Verification items for the finished model (mm, model axes). A direction names the side the tool comes from. Coordinates: 2 decimals unless noted, no trailing zeros. Loops run counter-clockwise (first coordinate to the right, second up) from the corner with the lowest first, then second, coordinate; pieces in that order, holes last. Notation, with made-up numbers: (-36.75, -23) - (-13.75, -23) arc R23 ccw to (-13.75, 1) - close; hole circle Ø6 at (6, 18). An arc over 180 degrees is marked (long way). Answer as CSV lines item,"result". Start each with the question number.
1. Gauge pin test, flat ends, axial feed: P1, Ø12.5, axis at y = 170, z = 0, coming from the -X side; P2, Ø5, axis at x = 5, z = -399, coming from the +Y side. Record the tip position at first contact, or that the pin passes through.
2. Material ranges on line 1 (Y direction, x = 4.5, z = 184); line 2 (Z direction, x = 7.75, y = 550); line 3 (Z direction, x = 0.5, y = 189.5), recorded low to high. Write a range as [from, to].
3. Release check for a two-part mould opening along Z. For faces 3 (the flat face through (0, 81, -130)), 4 (the flat face through (4.93, 261.39, -14.83)), 5 (the flat face through (4.93, 177.45, -246.5)) record: pulls with the +Z half, pulls with the -Z half, needs draft (parallel to the pull), parting line crosses it, or undercut.
4. Cross-section at C-C (z = -301). Enter the section's corners in (x, y), plus the area to 3 significant figures.
5. Cross-section at B-B (x = 1.75). State how many separate pieces and enclosed holes the cut face has, plus the area to 3 significant figures.
6. Set-up check for faces 1 (the flat face through (4.93, 63.37, 210.65)), 2 (the flat face through (10, 81, -130)): record each of +Z, -Z, +X, -X, +Y, -Y from which the full face is reachable in a straight line by a thin tool's end or side.
7. Cross-section at A-A (y = 251.5). Enter the section's corners in (x, z).
8. Cross-section at D-D (y = 489.5). Enter the section's corners in (x, z).
```python
from build123d import *

# Parameters (mm, degrees)
IZIM1_R                     = 152
IZIM1_R_2                   = 7
IZIM1_R_3                   = 13.5
IZIM1_R_4                   = 5.1
Y_KSEKLIK_EKSTR_ZYON1_DEPTH = 10


with BuildPart() as part:
    # Çizim1 → Yükseklik-Ekstrüzyon1 (new body)
    with BuildSketch(Plane(origin=(0, 0, 0), x_dir=(0, 0, -1), z_dir=(1, 0, 0))):
        Polygon((-250, 350), (-250, 570), (0, 570), (0, 350), (500, 0), (500, -200), (500, -240), (-250, -240), (-250, -200), align=None)
        Circle(IZIM1_R, mode=Mode.SUBTRACT)
        with Locations((0, 170)):
            Circle(IZIM1_R_2, mode=Mode.SUBTRACT)
        with Locations((99.92349289, 137.532889044)):
            Circle(IZIM1_R_2, mode=Mode.SUBTRACT)
        with Locations((161.67960777, 52.532889044)):
            Circle(IZIM1_R_2, mode=Mode.SUBTRACT)
        with Locations((161.67960777, -52.532889044)):
            Circle(IZIM1_R_2, mode=Mode.SUBTRACT)
        with Locations((99.92349289, -137.532889044)):
            Circle(IZIM1_R_2, mode=Mode.SUBTRACT)
        with Locations((0, -170)):
            Circle(IZIM1_R_2, mode=Mode.SUBTRACT)
        with Locations((-99.92349289, -137.532889044)):
            Circle(IZIM1_R_2, mode=Mode.SUBTRACT)
        with Locations((-161.67960777, -52.532889044)):
            Circle(IZIM1_R_2, mode=Mode.SUBTRACT)
        with Locations((-161.67960777, 52.532889044)):
            Circle(IZIM1_R_2, mode=Mode.SUBTRACT)
        with Locations((-99.92349289, 137.532889044)):
            Circle(IZIM1_R_2, mode=Mode.SUBTRACT)
        with Locations((-203.812062632, 211.374016696)):
            Circle(IZIM1_R_3, mode=Mode.SUBTRACT)
        with Locations((-183.812062632, 231.374016696)):
            Circle(IZIM1_R_4, mode=Mode.SUBTRACT)
        with Locations((-223.812062632, 231.374016696)):
            Circle(IZIM1_R_4, mode=Mode.SUBTRACT)
        with Locations((-183.812062632, 191.374016696)):
            Circle(IZIM1_R_4, mode=Mode.SUBTRACT)
        with Locations((-223.812062632, 191.374016696)):
            Circle(IZIM1_R_4, mode=Mode.SUBTRACT)
        with Locations((-210, 550)):
            Circle(IZIM1_R_2, mode=Mode.SUBTRACT)
        with Locations((-153.333333333, 550)):
            Circle(IZIM1_R_2, mode=Mode.SUBTRACT)
        with Locations((-96.666666667, 550)):
            Circle(IZIM1_R_2, mode=Mode.SUBTRACT)
        with Locations((-40, 550)):
            Circle(IZIM1_R_2, mode=Mode.SUBTRACT)
        with Locations((-210, -220)):
            Circle(IZIM1_R_2, mode=Mode.SUBTRACT)
        with Locations((-114.285714286, -220)):
            Circle(IZIM1_R_2, mode=Mode.SUBTRACT)
        with Locations((-18.571428571, -220)):
            Circle(IZIM1_R_2, mode=Mode.SUBTRACT)
        with Locations((77.142857143, -220)):
            Circle(IZIM1_R_2, mode=Mode.SUBTRACT)
        with Locations((172.857142857, -220)):
            Circle(IZIM1_R_2, mode=Mode.SUBTRACT)
        with Locations((268.571428571, -220)):
            Circle(IZIM1_R_2, mode=Mode.SUBTRACT)
        with Locations((364.285714286, -220)):
            Circle(IZIM1_R_2, mode=Mode.SUBTRACT)
        with Locations((460, -220)):
            Circle(IZIM1_R_2, mode=Mode.SUBTRACT)
        Polygon((29.246579563, 281.988117893), (0, 240.207289947), (9.011551126, 233.899204159), (38.258130688, 275.680032105), align=None, mode=Mode.SUBTRACT)
        Polygon((-200.681608906, 45.789510008), (-220.902149255, 81.456437938), (-230.471325041, 76.031414918), (-210.250784693, 40.364486987), align=None, mode=Mode.SUBTRACT)
    extrude(amount=Y_KSEKLIK_EKSTR_ZYON1_DEPTH)


solid = part.part
```
Values follow:
1,P1,"passes through"
1,P2,"stops at y = 72.45"
2,line 1,"y = [-240, 186.28], [196.47, 226.28], [236.47, 570]"
2,line 2,"z = [0, 33], [47, 89.67], [103.67, 146.33], [160.33, 203], [217, 250]"
2,line 3,"z = [-229.29, 179.07], [188.56, 219.07], [228.56, 250]"
3,face 3,"needs draft"
3,face 4,"undercut"
3,face 5,"pulls with the -Z half"
4,outline,"(0, -240) - (10, -240) - (10, 139.3) - (0, 139.3) - close"
4,area,"3,790 mm²"
5,separate pieces,"1"
5,enclosed holes,"30"
5,area,"332,000 mm²"
6,face 1,"+X, -X"
6,face 2,"+Z, -Z, +X, +Y, -Y"
7,outline,"(0, -140.71) - (10, -140.71) - (10, -21.33) - (0, -21.33) - close; (0, -7.9) - (10, -7.9) - (10, 250) - (0, 250) - close"
8,outline,"(0, 0) - (10, 0) - (10, 250) - (0, 250) - close"
